Geometry check sheet. Reference: the model listing, model coordinates, mm. Face numbers are marked on the shaded views. A direction names the side the tool comes from. Coordinates: 2 decimals unless noted, no trailing zeros. Loops run counter-clockwise (first coordinate to the right, second up) from the corner with the lowest first, then second, coordinate; pieces in that order, holes last. Notation, with made-up numbers: (86, -23.75) - (135, -23.75) arc R16 cw to (135, 0.25) - close; hole circle Ø6 at (60, -29.75). An arc over 180 degrees is marked (long way). One line per item, written item: value.
from build123d import *

# Parameters (mm, degrees)
F2_R     = 19.05
F3_DEPTH = 108.966
F4_R     = 6.35
F5_DEPTH = 115.316


with BuildPart() as f1:
    # F0 (on Top) → F1 (revolve)
    with BuildSketch(Plane.XY):
        Polygon((9.751909, 68.992269), (9.751909, 15.144269), (44.803909, 15.144269), (44.803909, 49.942269), (79.601909, 49.942269), (79.601909, 68.992269), align=None)
    revolve(axis=Axis((9.751909, 42.068269, 0), (0, 1, 0)))

    # F2 (on face) → F3 (cut)
    with BuildSketch(Plane.XZ.offset(-15.144269)):
        with Locations((9.751909, 0)):
            Circle(F2_R)
    extrude(amount=-F3_DEPTH, mode=Mode.SUBTRACT)

    # F4 (on face) → F5 (cut)
    with BuildSketch(Plane.XZ.offset(-49.942269)):
        with Locations((9.272376, 56.402412)):
            Circle(F4_R)
        with Locations((66.156359, 0)):
            Circle(F4_R)
        with Locations((-46.652542, 0)):
            Circle(F4_R)
        with Locations((9.751909, -56.404451)):
            Circle(F4_R)
    extrude(amount=-F5_DEPTH, mode=Mode.SUBTRACT)


solid = f1.part
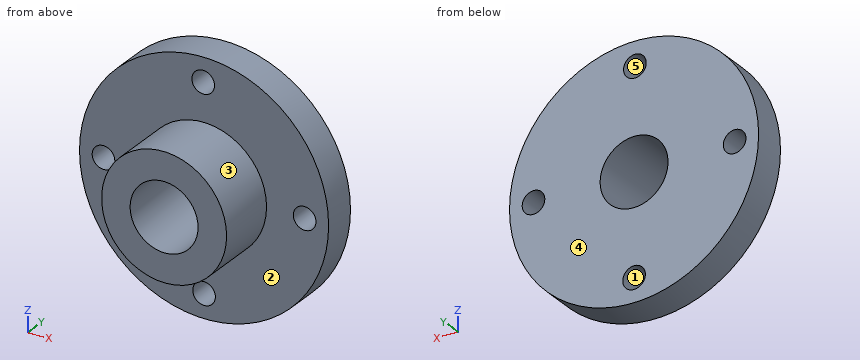
(1) Cross-section at D-D on y = 46.5. Record the cut outline in (x, z), and give its area (3 significant figures).
Reply:
outline: circle Ø70.1 at (9.75, 0); hole circle Ø38.1 at (9.75, 0)
area: 2,720 mm2
(2) Go/stop test with flat-tipped pins: pin 1 Ø7.5 at (x, z) = (-46.65, 0) entering from +Y; pin 2 Ø20.5 at (x, z) = (9.27, 56.4) entering from -Y; pin 3 Ø1.5 at (y, z) = (48.5, 4) entering from +X; pin 4 Ø12 at (x, y) = (-4, 55) entering from +Z. Record where each tip stops, or that it passes through.
Reply:
pin 1: through
pin 2: y = 49.94
pin 3: x = 44.65
pin 4: z = 69.42
(3) Release check for a two-part mould opening along X. For the marked faces 3, 4 and 5 record: pulls with the +X half, pulls with the -X half, needs draft (parallel to the pull), parting line crosses it, or undercut.
Reply:
face 3: parting line crosses it
face 4: needs draft
face 5: undercut
(4) Cross-section at A-A on z = 0. Record the cut outline in (x, y).
Reply:
outline: (-60.1, 49.94) - (-53, 49.94) - (-53, 68.99) - (-60.1, 68.99) - close; (-40.3, 49.94) - (-25.3, 49.94) - (-25.3, 15.14) - (-9.3, 15.14) - (-9.3, 68.99) - (-40.3, 68.99) - close; (28.8, 15.14) - (44.8, 15.14) - (44.8, 49.94) - (59.81, 49.94) - (59.81, 68.99) - (28.8, 68.99) - close; (72.51, 49.94) - (79.6, 49.94) - (79.6, 68.99) - (72.51, 68.99) - close
(5) Material ranges on probe 1 along Y at (x, z) = (7, 40.5); probe 2 along Z at (x, y) = (22, 59); probe 3 along Z at (x, y) = (23.5, 54.5), recorded low to high. Write a range as from..to.
Reply:
probe 1: 49.94..68.99
probe 2: -68.77..-14.59, 14.59..68.77
probe 3: -68.48..-13.19, 13.19..68.48
(6) Cross-section at B-B on x = 69.5. Record the cut outline in (y, z), and give its area (3 significant figures).
Reply:
outline: (49.94, -36.18) - (68.99, -36.18) - (68.99, -5.4) - (49.94, -5.4) - close; (49.94, 5.4) - (68.99, 5.4) - (68.99, 36.18) - (49.94, 36.18) - close
area: 1,170 mm2
(7) Access from +Z, -Z, +X, -X, +Y, -Y to the whole of each face (thin tool, end or side, straight path). Record for the marked faces 1 and 2.
Reply:
face 1: +Y, -Y
face 2: -Y
(8) Cross-section at C-C on x = 11. Record the cut outline in (y, z).
Reply:
outline: (15.14, -35.03) - (49.94, -35.03) - (49.94, -50.18) - (68.99, -50.18) - (68.99, -19.01) - (15.14, -19.01) - close; (15.14, 19.01) - (68.99, 19.01) - (68.99, 50.29) - (49.94, 50.29) - (49.94, 35.03) - (15.14, 35.03) - close; (49.94, -69.84) - (68.99, -69.84) - (68.99, -62.63) - (49.94, -62.63) - close; (49.94, 62.51) - (68.99, 62.51) - (68.99, 69.84) - (49.94, 69.84) - close
